Can you work these out from the model? Positions are in its coordinate system, mm. A direction names the side the tool comes from. Round coordinates to 2 decimals unless told otherwise and drop trailing zeros. Order: outer loops, then holes, each group sorted by start corner. A loop starts at its lowest first (then second) coordinate and runs counter-clockwise, first axis right, second up.
from build123d import *

# Parameters (mm, degrees)
SKETCH_1_R      = 4
EXTRUDE_1_DEPTH = 1.4


with BuildPart() as part:
    # Эскиз1 → Бобышка-Вытянуть1 (new, symmetric)
    with BuildSketch(Plane.XY):
        Polygon((39, -10), (44.6, -10), (44.6, -5), (47.4, -5), (47.4, 5), (44.6, 5), (44.6, 10), (39, 10), (39, 12.8), (31, 12.8), (31, 10), (21.5, 10), (21.5, 12.8), (13.5, 12.8), (13.5, 10), (4, 10), (4, 12.8), (-4, 12.8), (-4, 10), (-13.5, 10), (-13.5, 12.8), (-21.5, 12.8), (-21.5, 10), (-31, 10), (-31, 12.8), (-39, 12.8), (-39, 10), (-44.6, 10), (-44.6, 5), (-47.4, 5), (-47.4, -5), (-44.6, -5), (-44.6, -10), (-39, -10), (-39, -12.8), (-31, -12.8), (-31, -10), (-21.5, -10), (-21.5, -12.8), (-13.5, -12.8), (-13.5, -10), (-4, -10), (-4, -12.8), (4, -12.8), (4, -10), (13.5, -10), (13.5, -12.8), (21.5, -12.8), (21.5, -10), (31, -10), (31, -12.8), (39, -12.8), align=None)
        with Locations((20.5, 0)):
            Circle(SKETCH_1_R, mode=Mode.SUBTRACT)
        with Locations((-33.5, 0)):
            Circle(SKETCH_1_R, mode=Mode.SUBTRACT)
    extrude(amount=EXTRUDE_1_DEPTH, both=True)


solid = part.part
(1) I want a section at A-A, the plane y = 0. List the corners of the cut face in (x, z) for me.
(2) If we mould it in two halves opening along X, with no side actions, what happens to faces 4 (the face through (46, 5, 0)), 5 (the face through (4, 11, 0)), 6 (the face through (-44.6, 8, 0)), 7 (the face through (9, -10, 0))? For each: pulls with the +X half, pulls with the -X half, needs draft (parallel to the pull), parting line crosses it, or undercut.
(3) I want a section at C-C, the plane z = -0.65. Give the number of separate pieces and of enclosed holes in the cut face, plus the area to 3 significant figures.
(4) I want a section at D-D, the plane x = 18.5. List the corners of the cut face in (y, z) for me.
(5) I want a section at B-B, the plane x = -33.5. List the corners of the cut face in (y, z) for me, plus the area to 3 significant figures.
(6) I'm going to push flat-ended pins straight in: pin 1 Ø1.4 at (y, z) = (12, 0.5) entering from +X; pin 2 Ø1.4 at (x, z) = (-40.5, 0) entering from -Y; pin 3 Ø1.4 at (y, z) = (-11.5, 0) entering from -X. Where does each tip first touch, or does it pass through?
(7) Please list where these lines run through material, in increasing order: probe 1 along X at (y, z) = (3.5, 0.2); probe 2 along Y at (x, z) = (-33.5, -0.5); probe 3 along Y at (x, z) = (12, 0.8).
(8) On a 3-axis mill with a long thin cutter (end or side, diameter ignored), from which of +Z, -Z, +X, -X, +Y, -Y can I reach the whole of each face in a straight line? I mean faces 1 (the face through (39, -11, 0)), 2 (the face through (21.5, 11, 0)), 3 (the face through (-39, 11, 0)). Say none if no direction works.
Ans:
1. outline: (-47.4, -1.4) - (-37.5, -1.4) - (-37.5, 1.4) - (-47.4, 1.4) - close; (-29.5, -1.4) - (16.5, -1.4) - (16.5, 1.4) - (-29.5, 1.4) - close; (24.5, -1.4) - (47.4, -1.4) - (47.4, 1.4) - (24.5, 1.4) - close
2. face 4: needs draft
2. face 5: undercut
2. face 6: pulls with the -X half
2. face 7: undercut
3. separate pieces: 1
3. enclosed holes: 2
3. area: 1,960 mm2
4. outline: (-12.8, -1.4) - (-3.46, -1.4) - (-3.46, 1.4) - (-12.8, 1.4) - close; (3.46, -1.4) - (12.8, -1.4) - (12.8, 1.4) - (3.46, 1.4) - close
5. outline: (-12.8, -1.4) - (-4, -1.4) - (-4, 1.4) - (-12.8, 1.4) - close; (4, -1.4) - (12.8, -1.4) - (12.8, 1.4) - (4, 1.4) - close
5. area: 49.3 mm2
6. pin 1: stops at x = 39
6. pin 2: stops at y = -10
6. pin 3: stops at x = -39
7. probe 1: x = -47.4 to -35.44, -31.56 to 18.56, 22.44 to 47.4
7. probe 2: y = -12.8 to -4, 4 to 12.8
7. probe 3: y = -10 to 10
8. face 1: +Z, -Z, +X, -Y
8. face 2: +Z, -Z, +Y
8. face 3: +Z, -Z, -X, +Y
